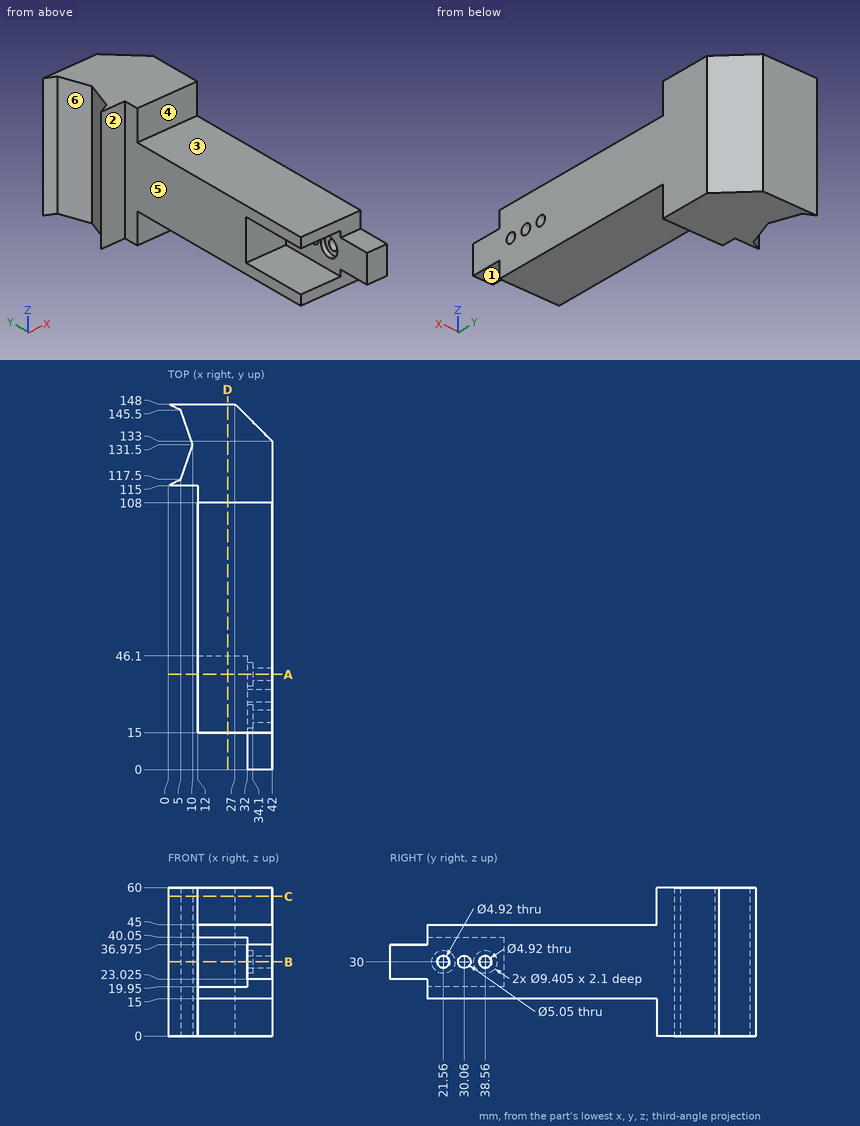
The drawing under review shows one solid part. Ordinate dimensions are in mm from its lowest x, y, z. A direction names the side the tool comes from. Round coordinates to 2 decimals unless told otherwise and drop trailing zeros. Order: outer loops, then holes, each group sorted by start corner. A loop starts at its lowest first (then second) coordinate and runs counter-clockwise, first axis right, second up. Notation, with made-up numbers: (18, 37) -> (55, 37) arc R17 cw to (55, 55) -> close; hole circle Ø4 at (80, 30.5). An arc over 180 degrees is marked (long way). Use a Markdown table: item, result.
Item 1: Draft analysis for pull direction Y (two halves, no side actions). For the marked faces 4, 5 and 6, state which applies: +Y half, -Y half, draft (parallel to the pull), parting line (faces both ways), or undercut.
Resolved:
| item | result |
|---|---|
| face 4 | -Y half |
| face 5 | draft |
| face 6 | undercut |
Item 2: Take a section at B-B (z = 30). State how many separate pieces and enclosed holes the cut face has, plus the area to 3 significant figures.
Resolved:
| item | result |
|---|---|
| separate pieces | 4 |
| enclosed holes | 0 |
| area | 3,410 mm² |
Item 3: Machinability: for the marked faces 1, 2 and 3, which of the approach directions +Z, -Z, +X, -X, +Y, -Y give a long, thin tool a straight path to every point of the face, cutting with its end or side? Answer none if there is none.
Resolved:
| item | result |
|---|---|
| face 1 | -Z, +X, -X, -Y |
| face 2 | +Z, -Z, -X, -Y |
| face 3 | +Z, +X, -X, -Y |
Item 4: Take a section at A-A (y = 38.56). State the section outline as (x, z) points, plus the area to 3 significant figures.
Resolved:
| item | result |
|---|---|
| outline | (12, 15) -> (42, 15) -> (42, 27.54) -> (34.1, 27.54) -> (34.1, 25.3) -> (32, 25.3) -> (32, 19.95) -> (12, 19.95) -> close; (12, 40.05) -> (32, 40.05) -> (32, 34.7) -> (34.1, 34.7) -> (34.1, 32.46) -> (42, 32.46) -> (42, 45) -> (12, 45) -> close |
| area | 439 mm² |
Item 5: Take a section at C-C (z = 56.5). State the section outline as (x, y) points, plus the area to 3 significant figures.
Resolved:
| item | result |
|---|---|
| outline | (0, 115) -> (12, 115) -> (12, 108) -> (42, 108) -> (42, 133) -> (27, 148) -> (0, 148) -> (5, 145.5) -> (10, 131.5) -> (5, 117.5) -> close |
| area | 1,260 mm² |
Item 6: Take a section at D-D (x = 24). State the section outline as (y, z) points.
Resolved:
| item | result |
|---|---|
| outline | (15, 15) -> (108, 15) -> (108, 0) -> (148, 0) -> (148, 60) -> (108, 60) -> (108, 45) -> (15, 45) -> (15, 40.05) -> (46.1, 40.05) -> (46.1, 19.95) -> (15, 19.95) -> close |
Item 7: For pin 1 (3 mm diameter, centred on y = 38, z = 28, fed in from -X); pin 2 (12 mm diameter, centred on x = 33, z = 9.5, fed in from -Y); pin 3 (5 mm diameter, centred on y = 75, z = 22, fed in from -X); pin 4 (8 mm diameter, centred on y = 30.06, z = 30, fed in from +X), all flat-tipped, find the tip position at first contact; note any pin that passes through.
Resolved:
| item | result |
|---|---|
| pin 1 | stops at x = 34.1 |
| pin 2 | stops at y = 15 |
| pin 3 | stops at x = 12 |
| pin 4 | stops at x = 42 |
Item 8: For line 1 along Z through (x, y) = (39.25, 38.56); line 2 along Y through (x, z) = (33.7, 30) (1 decimal); line 3 along Y through (x, z) = (37.25, 30) (3 decimals), list the stretches that pass through material, from the lowest coordinate up. Write a range as [from, to].
Resolved:
| item | result |
|---|---|
| line 1 | z = [15, 27.54], [32.46, 45] |
| line 2 | y = [0, 16.9], [26.3, 27.5], [32.6, 33.9], [43.3, 141.3] |
| line 3 | y = [0, 19.1], [24.02, 27.535], [32.585, 36.1], [41.02, 137.75] |
